Solid Edge part; units mm, degrees
sketch "Sketch1" plane through (0, 0, 0) normal (0, 0, 1) x (1, 0, 0)
  circle A0 centre (-27.5, 16) radius 5
  line L0 (37.5, 26) -> (-37.5, 26)
  line L1 (-37.5, 26) -> (-37.5, -26)
  line L2 (-37.5, -26) -> (37.5, -26)
  line L3 (37.5, -26) -> (37.5, 26)
  circle A1 centre (27.5, -16) radius 5
  circle A2 centre (27.5, 16) radius 5
  circle A3 centre (-27.5, -16) radius 5
extrude "Protrusion1" add sketch "Sketch1" against normal blind 15
sketch "Sketch2" plane through (0, 0, 0) normal (0, 0, 1) x (1, 0, 0)
  line L0 (-12.5, 6) -> (-32.5, 6)
  line L1 (-32.5, 6) -> (-32.5, -6)
  line L2 (-32.5, -6) -> (-12.5, -6)
  line L3 (-12.5, -6) -> (-12.5, 6)
extrude "ExtrudedProtrusion_2" add sketch "Sketch2" along normal blind 10
sketch "Sketch3" plane through (-22.5, -6, 5) normal (0, -1, 0) x (1, 0, 0)
  line L0 (20, 15) -> (20, 35)
  line L1 (10, 5) -> (-10, 5)
  arc A0 (-10, 5) -> (20, 35) centre (20, 5) cw
  arc A1 (10, 5) -> (20, 15) centre (20, 5) cw
extrude "ExtrudedProtrusion_3" add sketch "Sketch3" against normal blind 12
sketch "Sketch4" plane through (-2.5, 0, 30) normal (1, 0, 0) x (0, 1, 0)
  line L0 (6, 10) -> (6, -10)
  line L1 (6, -10) -> (-6, -10)
  line L2 (-6, -10) -> (-6, 10)
  line L3 (-6, 10) -> (6, 10)
extrude "ExtrudedProtrusion_4" add sketch "Sketch4" along normal blind 10
sketch "Sketch5" plane through (2.5, 0, 40) normal (0, 0, 1) x (1, 0, 0)
  line L0 (5, 6) -> (5, -6)
  arc A0 (5, 6) -> (5, -6) centre (20, 0) cw
  circle A1 centre (20, 0) radius 8
extrude "Protrusion2" add sketch "Sketch5" against normal up to vertex (20 mm away)
Can you work these out from the model? Positions are in its coordinate system, mm. A direction names the side the tool comes from. Coordinates: 2 decimals unless noted, no trailing zeros. Write each loop counter-clockwise with the first axis right and the second up, starting at its lowest first coordinate (ties: lowest second). Pieces come first, ordered by that corner, then holes. Notation, with made-up numbers: M -30,18 L -14,18 A33 ccw -14,57 Z; hole C 2.25,-11 d11. An arc over 180 degrees is marked long. Use one line per item in the form item = value.
Q1. If we section it at B-B (x = -27.5): Write out the boundary of the cut face in (y, z).
Model answer:
outline = M -26,-15 L -21,-15 L -21,0 L -26,0 Z; M -11,-15 L 11,-15 L 11,0 L 6,0 L 6,26.58 L -6,26.58 L -6,0 L -11,0 Z; M 21,-15 L 26,-15 L 26,0 L 21,0 Z
Q2. If we section it at C-C (z = 34): Write out the boundary of the cut face in (x, y), then the cut area to 3 significant figures.
Model answer:
outline = M -20.5,-6 L 7.5,-6 A16.16 ccw long 7.5,6 L -20.5,6 Z; hole C 22.5,0 d16
area = 946 mm^2
Q3. For P1, Ø10, axis at y = -6.5, z = 26.5, coming from the -X side; P2, Ø11, axis at y = 3, z = 7, coming from the -X side; P3, Ø8, axis at y = -12.5, z = 23, coming from the -X side, each with a flat end and sliding along its axis, tell me the tip position at first contact or that it passes through.
Model answer:
P1 = -30.2
P2 = -32.5
P3 = 8.76
Q4. For faces 1 (the cylindrical face through (-9.49, -0.08, 17.15)), 2 (the flat face through (37.5, 0, -7)), 3 (the flat face through (-13, -6, 20)), which set-ups out of +Z, -Z, +X, -X, +Y, -Y let a thin tool reach every point of the face, with its end or its side?
Model answer:
face_1 = +X, +Y, -Y
face_2 = -Z, +X, +Y, -Y
face_3 = +Z, -X, -Y
Q5. We'd pull the mould along X, two halves only. Please class faces 4 (the flat face through (-32.5, 0, 5)), 5 (the cylindrical face through (38.643, -0.624, 30.14)), 6 (the cylindrical face through (-31.5, 13, -7.4)), 7 (the cylindrical face through (23.5, 13, -7.4)): +X half, -X half, draft (parallel to the pull), parting line (faces both ways), or undercut.
Model answer:
face_4 = -X half
face_5 = parting line
face_6 = undercut
face_7 = undercut
Q6. If we section it at D-D (x = 27.5): Write out the boundary of the cut face in (y, z) (3 decimals), then the cut area to 3 significant figures.
Model answer:
outline = M -26,-15 L -21,-15 L -21,0 L -26,0 Z; M -15.362,20 L -6.245,20 L -6.245,40 L -15.362,40 Z; M -11,-15 L 11,-15 L 11,0 L -11,0 Z; M 6.245,20 L 15.362,20 L 15.362,40 L 6.245,40 Z; M 21,-15 L 26,-15 L 26,0 L 21,0 Z
area = 845 mm^2
Q7. If we section it at A-A (y = 0): Write out the boundary of the cut face in (x, z).
Model answer:
outline = M -37.5,-15 L 37.5,-15 L 37.5,0 L -12.5,0 L -12.5,10 A10 cw -2.5,20 L 14.5,20 L 14.5,40 L -2.5,40 A30 ccw -32.5,10 L -32.5,0 L -37.5,0 Z; M 30.5,20 L 38.66,20 L 38.66,40 L 30.5,40 Z
Q8. I need wall thicknesses on line 1 along Y through (x, z) = (27.5, -11.25); line 2 along Y through (x, z) = (22.5, 34); line 3 along Z through (x, y) = (23.5, 9). Which ranges of each line are inside material? Lowest first, please. Write a range as from..to.
Model answer:
line_1 = -26..-21, -11..11, 21..26
line_2 = -16.16..-8, 8..16.16
line_3 = -15..0, 20..40
